Input: part model. Units: mm. Frame: model coordinates. A direction names the side the tool comes from. Coordinates: 2 decimals unless noted, no trailing zeros. Write each loop counter-clockwise with the first axis right and the second up, starting at its lowest first coordinate (ties: lowest second). Pieces come first, ordered by that corner, then holes. Notation, with made-up numbers: M 36,82.5 L 47,82.5 A32 ccw 47,119.5 Z; hole C -24.75,26.25 d5. An arc over 180 degrees is marked long. Write each question's results on one line, items separated by ' | '. Start each with the question number.
1. Section query D-D, the plane x = -10. Output: boundary loops of the cut face in (y, z).
2. Pull-direction query (X, two-part tool) for faces 1 (the flat face through (-20, 4, -30)), 2 (the flat face through (39.4, 0, -6.9)), 3 (the flat face through (38, 7, -9.9)), 4 (the cylindrical face through (-10, 6, -8)); classes: +X half, -X half, draft (parallel to the pull), parting line (faces both ways), or undercut.
3. First-contact query: pin 1 (3.5 mm diameter, centred on x = 37, y = 6, fed in from -Z); pin 2 (3 mm diameter, centred on x = 0.5, z = -8.5, fed in from -Y); pin 3 (3.5 mm diameter, centred on x = 6.5, z = -7, fed in from +Y); pin 4 (1.8 mm diameter, centred on x = 28.5, z = -9, fed in from -Y). Flat tips, straight axial feed; report the tip coordinate or a pass-through.
4. Section query B-B, the plane x = 6.5. Output: boundary loops of the cut face in (y, z).
5. Ray query, probe 1 along Z at (x, y) = (-10, 6.4); probe 2 along Z at (x, y) = (-10, 1.2); probe 3 along Z at (x, y) = (37.5, 1.1). Return the intervals inside material, ascending.
6. Section query A-A, the plane y = 1.5. Output: boundary loops of the cut face in (x, z), and give its area (3 significant figures).
7. Set-up query: faces 5 (the flat face through (-8, 3, -11)), 6 (the cylindrical face through (7.7, 2.5, -7.9)), 7 (the flat face through (40.023, 6.521, -8.43)), 8 (the flat face through (28, 3, -7)). Return all of +Z, -Z, +X, -X, +Y, -Y with unobstructed straight access to the full face (end or side cutting, diameter ignored); none if empty.
8. Section query C-C, the plane z = -50. Output: boundary loops of the cut face in (x, y), and give its area (3 significant figures).
```python
from build123d import *

# Parameters (mm, degrees)
F1_DEPTH = 14
F0_W     = 20
F0_H     = 8
F2_DEPTH = 60
F3_R     = 4
F3_R_2   = 2
F3_R_3   = 1.5
F4_DEPTH = 8.001
F5_DEPTH = 3
F6_DEPTH = 5


# Not quite as in the source:
# - a feature names something its author has since deleted; it is built from what else it names


with BuildPart() as f1:
    # F0 (on Top) → F1 (new body)
    with BuildSketch(Plane.XY):
        Polygon((43, 0), (43, 8), (0, 8), (0, 0), (22, 0), (25, 3), (31, 3), (34, 0), align=None)
    extrude(amount=-F1_DEPTH)

    # F0 (on Top) → F2 (join)
    with BuildSketch(Plane.XY):
        with Locations((-10, 4)):
            Rectangle(F0_W, F0_H)
    extrude(amount=-F2_DEPTH)

    # F3 (on face) → F4 (cut, through all)
    with BuildSketch(Plane(origin=(0, 8, 0), x_dir=(-1, 0, 0), z_dir=(0, 1, 0))):
        with Locations((10, -10)):
            Circle(F3_R)
        with Locations((10, -10)):
            Circle(F3_R_2, mode=Mode.SUBTRACT)
        with Locations((10, -50)):
            Circle(F3_R)
        with Locations((10, -50)):
            Circle(F3_R_2, mode=Mode.SUBTRACT)
        with Locations((10, -10)):
            Circle(F3_R_2)
        with Locations((10, -50)):
            Circle(F3_R_2)
        with Locations((-37.5, -7)):
            Circle(F3_R_3)
        with Locations((-6.5, -7)):
            Circle(F3_R_3)
    extrude(amount=-F4_DEPTH, mode=Mode.SUBTRACT)

    # F3 (on face) → F5 (cut)
    with BuildSketch(Plane(origin=(0, 8, 0), x_dir=(-1, 0, 0), z_dir=(0, 1, 0))):
        Polygon((-8.1743157806, -9.9), (-4.8256842194, -9.9), (-3.1513684387, -7), (-4.8256842194, -4.1), (-8.1743157806, -4.1), (-9.8486315613, -7), align=None)
        with Locations((-6.5, -7)):
            Circle(F3_R_3, mode=Mode.SUBTRACT)
        Polygon((-39.1743157806, -9.9), (-35.8256842194, -9.9), (-34.1513684387, -7), (-35.8256842194, -4.1), (-39.1743157806, -4.1), (-40.8486315613, -7), align=None)
        with Locations((-37.5, -7)):
            Circle(F3_R_3, mode=Mode.SUBTRACT)
    extrude(amount=-F5_DEPTH, mode=Mode.SUBTRACT)

    # F3 (on face) → F6 (join)
    with BuildSketch(Plane(origin=(0, 8, 0), x_dir=(-1, 0, 0), z_dir=(0, 1, 0))):
        with Locations((10, -10)):
            Circle(F3_R)
        with Locations((10, -10)):
            Circle(F3_R_2, mode=Mode.SUBTRACT)
        with Locations((10, -50)):
            Circle(F3_R)
        with Locations((10, -50)):
            Circle(F3_R_2, mode=Mode.SUBTRACT)
    extrude(amount=-F6_DEPTH)


solid = f1.part
```
Answer:
1) outline: M 0,-60 L 8,-60 L 8,-52 L 3,-52 L 3,-54 L 0,-54 Z; M 0,-46 L 3,-46 L 3,-48 L 8,-48 L 8,-12 L 3,-12 L 3,-14 L 0,-14 Z; M 0,-6 L 3,-6 L 3,-8 L 8,-8 L 8,0 L 0,0 Z
2) face 1: -X half | face 2: draft | face 3: undercut | face 4: undercut
3) pin 1: z = -14 | pin 2: y = 0 | pin 3: y = 5 | pin 4: y = 3
4) outline: M 0,-14 L 8,-14 L 8,-9.9 L 5,-9.9 L 5,-8.5 L 0,-8.5 Z; M 0,-5.5 L 5,-5.5 L 5,-4.1 L 8,-4.1 L 8,0 L 0,0 Z
5) probe 1: -60 to -52, -48 to -12, -8 to 0 | probe 2: -60 to -54, -46 to -14, -6 to 0 | probe 3: -14 to -8.5, -5.5 to 0
6) outline: M -20,-60 L 0,-60 L 0,-14 L 23.5,-14 L 23.5,0 L -20,0 Z; M 32.5,-14 L 43,-14 L 43,0 L 32.5,0 Z; hole C -10,-50 d8; hole C -10,-10 d8; hole C 6.5,-7 d3; hole C 37.5,-7 d3 | area: 1,560 mm^2
7) face 5: -Y | face 6: +Y, -Y | face 7: +Y | face 8: +Z, -Z, -Y
8) outline: M -20,0 L -14,0 L -14,3 L -12,3 L -12,8 L -20,8 Z; M -8,3 L -6,3 L -6,0 L 0,0 L 0,8 L -8,8 Z | area: 116 mm^2
